Autodesk Inventor part; units mm, degrees
ref_plane "XZ Plane" through (0, 0, 0) normal (0, 1, 0) x (-1, 0, 0)
ref_plane "XY Plane" through (0, 0, 0) normal (0, 0, 1) x (1, 0, 0)
sketch "Sketch1" plane through (0, 0, 0) normal (0, 0, 1) x (1, 0, 0)
  line L0 (-37.75, 2.75) -> (37.75, 2.75)
  line L1 (37.75, 2.75) -> (37.75, -2.75)
  line L2 (37.75, -2.75) -> (-37.75, -2.75)
  line L3 (-37.75, -2.75) -> (-37.75, 2.75)
  point P0 (0, 0)
  point P1 (0, 2.75)
  point P2 (-37.75, 0)
  dimension "d0" = 5.5
  dimension "d1" = 75.5
extrude "Extrusion1" add sketch "Sketch1" along normal mid plane 103.5
ref_plane "Work Plane1" through (0, 0, 0) normal (1, 0, 0) x (0, 1, 0)
sketch "Sketch6" plane through (0, 0, 0) normal (1, 0, 0) x (0, 1, 0)
  line L0 (-2.75, 51.75) -> (-2.75, -51.75)
  line L1 (-2.75, 49.5) -> (-4.75, 48.3453)
  line L2 (-4.75, 48.3453) -> (-4.75, 47.6547)
  line L3 (-4.75, 47.6547) -> (-2.75, 46.5)
  line L4 (-2.75, 46.5) -> (-2.75, 49.5)
  point P0 (0, 0)
  point P1 (-2.75, 48)
  point P2 (-4.75, 48)
  dimension "d17" = 2.25
  dimension "d18" = 3
  dimension "d19" = 2
  dimension "d20" = 60
extrude "Extrusion4" add sketch "Sketch6" along normal mid plane 59.9
sketch "Sketch7" plane through (-37.75, 2.75, 51.75) normal (0, 1, 0) x (1, 0, 0)
  line L0 (75.5, 0) -> (0, 0)
  line L1 (44.3814, 15) -> (44.3814, 5)
  line L2 (44.3814, 5) -> (31.1186, 5)
  line L3 (31.1186, 5) -> (31.1186, 15)
  arc A0 (44.3814, 15) -> (31.1186, 15) centre (37.75, 15) ccw
  point P0 (37.75, 51.75)
  point P1 (37.75, 5)
  point P2 (37.75, 0)
  point P3 (37.75, 0)
  dimension "d23" = 5
  dimension "d25" = 10
  dimension "d26" = 6.6314
extrude "Extrusion5" cut sketch "Sketch7" against normal blind 2
chamfer "Chamfer2" distance 1 angle 45 4 edges at (0, 2.75, 30.1186) (6.6314, 2.75, 41.75) (-6.6314, 2.75, 41.75) (0, 2.75, 46.75)
sketch "Sketch8" plane through (-37.75, 2.75, 51.75) normal (0, 1, 0) x (1, 0, 0)
  line L0 (0, 103.5) -> (75.5, 103.5)
  line L1 (3, 100.5) -> (72.5, 100.5)
  line L2 (72.5, 100.5) -> (72.5, 6)
  line L3 (72.5, 6) -> (3, 6)
  line L4 (3, 6) -> (3, 100.5)
  line L5 (0, 103.5) -> (0, 0)
  line L6 (75.5, 0) -> (0, 0)
  line L7 (9.25, 96.25) -> (66.25, 96.25)
  line L8 (66.25, 96.25) -> (66.25, 10.25)
  line L9 (66.25, 10.25) -> (9.25, 10.25)
  line L10 (9.25, 10.25) -> (9.25, 96.25)
  line L11 (18.25, 71.25) -> (44.25, 71.25)
  line L12 (44.25, 71.25) -> (44.25, 18.25)
  line L13 (44.25, 18.25) -> (18.25, 18.25)
  line L14 (18.25, 18.25) -> (18.25, 71.25)
  line L15 (18.25, 44.75) -> (44.25, 44.75)
  line L16 (18.25, 58) -> (44.25, 58)
  line L17 (18.25, 31.5) -> (44.25, 31.5)
  circle A0 centre (24.75, 58) radius 3
  circle A1 centre (24.75, 44.75) radius 3
  circle A2 centre (24.75, 31.5) radius 3
  circle A3 centre (37.75, 58) radius 3
  circle A4 centre (37.75, 44.75) radius 3
  circle A5 centre (37.75, 31.5) radius 3
  point P0 (37.75, 51.75)
  point P1 (37.75, 100.5)
  point P2 (37.75, 103.5)
  point P3 (37.75, 96.25)
  point P4 (3, 53.25)
  point P5 (9.25, 53.25)
  point P6 (31.25, 31.5)
  dimension "d32" = 3
  dimension "d33" = 3
  dimension "d34" = 6
  dimension "d35" = 57
  dimension "d36" = 86
  dimension "d37" = 8
  dimension "d38" = 53
  dimension "d39" = 26
  dimension "d40" = 22
  dimension "d44" = 6.5
  dimension "d45" = 6.5
  dimension "d46" = 6.5
  dimension "d47" = 6.5
  dimension "d48" = 6.5
  dimension "d49" = 6.5
  dimension "d50" = 6
  dimension "d51" = 6
  dimension "d52" = 6
  dimension "d53" = 6
  dimension "d54" = 6
  dimension "d55" = 6
  dimension "d56" = 13.25
  dimension "d57" = 26.5
  dimension "d58" = 13.25
extrude "Extrusion6" cut sketch "Sketch8" against normal up to surface (5.5 mm away) contours A0 L16 | L16 A0 | A3 L16 | L16 A3 | A1 L15 | L15 A1 | A4 L15 | L15 A4 | A2 L17 | L17 A2 | A5 L17 | L17 A5
chamfer "Chamfer3" distance 0.5 angle 45 6 edges at (-16, 2.75, -6.25) (-16, 2.75, 7) (-16, 2.75, 20.25) (-3, 2.75, 20.25) (-3, 2.75, 7) (-3, 2.75, -6.25)
Geometry: final body of the model. Coordinates: model frame, mm. A direction names the side the tool comes from. Round coordinates to 2 decimals unless told otherwise and drop trailing zeros. Loops run counter-clockwise (first coordinate to the right, second up) from the corner with the lowest first, then second, coordinate; pieces in that order, holes last. Notation, with made-up numbers: (60.5, 5) - (76.5, 5) arc R17 cw to (76.5, 30) - close; hole circle Ø9 at (12.5, 77.25). An arc over 180 degrees is marked (long way). Write each question's results on one line, items separated by ' | '. Start each with the question number.
1) Line query: probe 1 along X at (y, z) = (0.5, -6.25); probe 2 along Z at (x, y) = (0, 0.6); probe 3 along Z at (x, y) = (0, 0.9). Output: solid intervals per line, ascending. Write a range as [from, to].
2) First-contact query: P1, Ø2, axis at y = -4, z = 47.5, coming from the +X side; P2, Ø2, axis at x = 3, z = -35.5, coming from the -Y side; P3, Ø5.5, axis at x = -13, z = 7, coming from the -Y side; P4, Ø1, axis at y = -3.5, z = 48.5, coming from the -X side. Flat tips, straight axial feed; report the tip coordinate or a pass-through.
3) Cut plane C-C on x = -25. Return loops of the section in (y, z), then the cut area to 3 significant figures.
4) Cut plane D-D on z = -31. Return loops of the section in (x, y).
5) Mould query, pull axis Z, two halves, no side actions, for faces 4 (the face through (-1, 0, -51.75)), 5 (the face through (-15.21, -0.21, 4.97)), 6 (the face through (-1, 2.75, -1)), 7 (the face through (0.15, 1.26, 30.12)). Classes: released by +Z, released by -Z, zero draft, split by the parting line, or undercut.
6) Cut plane A-A on x = 0. Count the separate pieces of the cut face and the enclosed holes in it, then the cut area to 3 significant figures.
7) Cut plane B-B on z = 7. Return loops of the section in (x, y), then the cut area to 3 significant figures.
8) Access query for faces 1 (the face through (29.95, -4, 48)), 2 (the face through (-29.95, -4, 48)), 3 (the face through (0, 0.75, 38)). Directions: +Z, -Z, +X, -X, +Y, -Y. A direction counts if a zero-diameter tool reaches every point of the face in a straight line with its end or side. Return the directions, or none.
Verdict:
1) probe 1: x = [-37.75, -16], [-10, -3], [3, 37.75] | probe 2: z = [-51.75, -9.25], [-3.25, 4], [10, 17.25], [23.25, 51.75] | probe 3: z = [-51.75, -9.25], [-3.25, 4], [10, 17.25], [23.25, 30.12], [46.75, 51.75]
2) P1: stops at x = 29.95 | P2: stops at y = -2.75 | P3: passes through | P4: stops at x = -29.95
3) outline: (-4.75, 47.65) - (-2.75, 46.5) - (-2.75, -51.75) - (2.75, -51.75) - (2.75, 51.75) - (-2.75, 51.75) - (-2.75, 49.5) - (-4.75, 48.35) - close | area: 573 mm2
4) outline: (-37.75, -2.75) - (37.75, -2.75) - (37.75, 2.75) - (-37.75, 2.75) - close
5) face 4: released by -Z | face 5: undercut | face 6: zero draft | face 7: undercut
6) separate pieces: 4 | enclosed holes: 0 | area: 439 mm2
7) outline: (-37.75, -2.75) - (-16, -2.75) - (-16, 2.25) - (-16.5, 2.75) - (-37.75, 2.75) - close; (-10, -2.75) - (-3, -2.75) - (-3, 2.25) - (-3.5, 2.75) - (-9.5, 2.75) - (-10, 2.25) - close; (3, -2.75) - (37.75, -2.75) - (37.75, 2.75) - (3.5, 2.75) - (3, 2.25) - close | area: 349 mm2
8) face 1: +Z, -Z, +X, -Y | face 2: +Z, -Z, -X, -Y | face 3: +Y
